```python
from build123d import *

# Parameters (mm, degrees)
SKETCH4_W           = 8
SKETCH4_H           = 5
EXTRUDE1_DEPTH      = 19.1
SKETCH6_W           = 17.706910835
SKETCH6_H           = 1.662230216
CUT_EXTRUDE1_DEPTH  = 18.6
SKETCH7_W           = 17.592020929
SKETCH7_H           = 1.332722913
CUT_EXTRUDE2_DEPTH  = 18.6
SKETCH8_W           = 5.300719424
SKETCH8_H           = 17.765707434
SKETCH8_W_2         = 2.943884892
SKETCH8_H_2         = 17.795443645
CUT_EXTRUDE3_DEPTH  = 18.6
SKETCH10_W          = 3.9
SKETCH10_H          = 17.990453763
CUT_EXTRUDE4_DEPTH  = 2
SKETCH11_R          = 0.25
CUT_EXTRUDE5_DEPTH  = 2
CUT_EXTRUDE6_DEPTH  = 2
SKETCH14_R          = 0.35
CUT_EXTRUDE8_DEPTH  = 2
CUT_EXTRUDE16_DEPTH = 2.6
CUT_EXTRUDE16_DRAFT = 3.5
SKETCH29_W          = 8
SKETCH29_H          = 5
SKETCH29_W_2        = 6
SKETCH29_H_2        = 4.3
CUT_EXTRUDE19_DEPTH = 2.5
CUT_EXTRUDE20_DEPTH = 5.3
CUT_EXTRUDE21_DEPTH = 7
SKETCH19_R          = 1
CUT_EXTRUDE11_DEPTH = 11.25


with BuildPart() as part:
    # Sketch4 → Extrude1 (new body)
    with BuildSketch(Plane.XY):
        with Locations((-4, 2.5)):
            Rectangle(SKETCH4_W, SKETCH4_H)
    extrude(amount=EXTRUDE1_DEPTH)

    # Sketch6 → Cut-Extrude1 (cut)
    with BuildSketch(Plane(origin=(0, 0, 0), x_dir=(0, 0, -1), z_dir=(1, 0, 0))):
        with Locations((-10.453455418, -0.081115108)):
            Rectangle(SKETCH6_W, SKETCH6_H)
    extrude(amount=-CUT_EXTRUDE1_DEPTH, mode=Mode.SUBTRACT)

    # Sketch7 → Cut-Extrude2 (cut)
    with BuildSketch(Plane(origin=(0, 0, 0), x_dir=(0, 0, -1), z_dir=(1, 0, 0))):
        with Locations((-10.396010465, 4.916361457)):
            Rectangle(SKETCH7_W, SKETCH7_H)
    extrude(amount=-CUT_EXTRUDE2_DEPTH, mode=Mode.SUBTRACT)

    # Sketch8 → Cut-Extrude3 (cut)
    with BuildSketch(Plane.XZ.offset(-0.75)):
        with Locations((-9.250359712, 10.482853717)):
            Rectangle(SKETCH8_W, SKETCH8_H)
        with Locations((0.071942446, 10.497721823)):
            Rectangle(SKETCH8_W_2, SKETCH8_H_2)
    extrude(amount=-CUT_EXTRUDE3_DEPTH, mode=Mode.SUBTRACT)

    # Sketch10 → Cut-Extrude4 (cut)
    with BuildSketch(Plane(origin=(0, 4.25, 0), x_dir=(1, 0, 0), z_dir=(0, 1, 0))):
        with Locations((-4, -10.595226882)):
            Rectangle(SKETCH10_W, SKETCH10_H)
    extrude(amount=-CUT_EXTRUDE4_DEPTH, mode=Mode.SUBTRACT)

    # Sketch11 → Cut-Extrude5 (cut)
    with BuildSketch(Plane(origin=(0, 2.25, 0), x_dir=(1, 0, 0), z_dir=(0, 1, 0))):
        with Locations(Location((-3.85, -11.2, 0), (0, 0, 270))):  # turned: the seam where the file's is
            Circle(SKETCH11_R)
    extrude(amount=-CUT_EXTRUDE5_DEPTH, mode=Mode.SUBTRACT)

    # Sketch12 → Cut-Extrude6 (cut)
    with BuildSketch(Plane(origin=(0, 2.25, 0), x_dir=(1, 0, 0), z_dir=(0, 1, 0))):
        with BuildLine():
            Line((-3.2, -19.099584714), (-3.2, -11.099584714))
            ThreePointArc((-3.2, -11.099584714), (-2.95, -10.849584714), (-2.7, -11.099584714))
            Line((-2.7, -11.099584714), (-2.7, -19.099584714))
            ThreePointArc((-2.7, -19.099584714), (-2.95, -19.349584714), (-3.2, -19.099584714))
        make_face()
    extrude(amount=-CUT_EXTRUDE6_DEPTH, mode=Mode.SUBTRACT)

    # Sketch14 → Cut-Extrude8 (cut)
    with BuildSketch(Plane(origin=(0, 2.25, 0), x_dir=(1, 0, 0), z_dir=(0, 1, 0))):
        with Locations(Location((-4.95, -1.975, 0), (0, 0, 270))):  # turned: the seam where the file's is
            Circle(SKETCH14_R)
    extrude(amount=-CUT_EXTRUDE8_DEPTH, mode=Mode.SUBTRACT)


with BuildPart() as cut_extrude16_tool:
    # Sketch28 → Cut-Extrude16 (with draft: the straight prism first)
    with BuildSketch(Plane.XY.offset(1.6)):
        with BuildLine():
            ThreePointArc((-3.25, 3.1), (-3, 2.85), (-2.75, 3.1))
            Line((-2.75, 3.1), (-2.75, 5))
            Line((-2.75, 5), (-3.25, 5))
            Line((-3.25, 5), (-3.25, 3.1))
        make_face()
    extrude(amount=-CUT_EXTRUDE16_DEPTH)
    # Cut-Extrude16: the draft: its side faces are tilted about the plane it starts from
    cut_extrude16_sides = [cut_extrude16_tool.faces().sort_by_distance(p)[0] for p in [
        (-3, 2.85, 0.3),
        (-2.75, 4.05, 0.3),
        (-3, 5, 0.3),
        (-3.25, 4.05, 0.3),
    ]]
    draft(cut_extrude16_sides, Plane.XY.offset(1.6), CUT_EXTRUDE16_DRAFT)


with BuildPart() as part_1:
    add(part.part)

    # Cut-Extrude16: cut by cut_extrude16_tool
    add(cut_extrude16_tool.part, mode=Mode.SUBTRACT)

    # Sketch29 → Cut-Extrude19 (cut)
    with BuildSketch(Plane.XY.offset(1.6)):
        with Locations((-4, 2.5)):
            Rectangle(SKETCH29_W, SKETCH29_H)
        with Locations((-4, 2.5)):
            Rectangle(SKETCH29_W_2, SKETCH29_H_2, mode=Mode.SUBTRACT)
    extrude(amount=-CUT_EXTRUDE19_DEPTH, mode=Mode.SUBTRACT)

    # Sketch18 → Cut-Extrude20 (cut, through all)
    with BuildSketch(Plane(origin=(0, 4.65, 0), x_dir=(1, 0, 0), z_dir=(0, 1, 0))):
        Polygon((-3.8, 0), (-7, -0.85), (-7, 0), align=None)
        Polygon((-2.2, 0), (-1, 0), (-1, -0.85), align=None)
    extrude(amount=-CUT_EXTRUDE20_DEPTH, mode=Mode.SUBTRACT)

    # Sketch30 → Cut-Extrude21 (cut, through all)
    with BuildSketch(Plane.ZY.offset(7)):
        Polygon((0, 3.9), (0.85, 4.65), (0, 4.65), align=None)
        Polygon((0, 2.3), (0.85, 0.35), (0, 0.35), align=None)
    extrude(amount=-CUT_EXTRUDE21_DEPTH, mode=Mode.SUBTRACT)

    # Sketch19 → Cut-Extrude11 (cut)
    with BuildSketch(Plane.XY.offset(1.6)):
        with Locations((-4.85, 3.1)):
            Circle(SKETCH19_R)
    extrude(amount=CUT_EXTRUDE11_DEPTH, mode=Mode.SUBTRACT)


solid = part_1.part
```
The listing builds one solid part. Answer for the finished solid, in the listing's coordinates (mm). A direction names the side the tool comes from. Round coordinates to 2 decimals unless told otherwise and drop trailing zeros. Order: outer loops, then holes, each group sorted by start corner. A loop starts at its lowest first (then second) coordinate and runs counter-clockwise, first axis right, second up. Notation, with made-up numbers: (15.5, 50.5) -> (45.5, 50.5) arc R24 cw to (45.5, 63.5) -> close; hole circle Ø7 at (63.5, -37.5). An arc over 180 degrees is marked (long way). Answer as CSV lines item,"result". Start each with the question number.
(1) Find the intervals of material crossed by probe 1 along X at (y, z) = (4.2, 7.5); probe 2 along X at (y, z) = (1.6, 11.2); probe 3 along X at (y, z) = (1, 17.25), in increasing order. Write a range as from..to.
(2) A tool of negligible diameter and unlimited length cuts with its end or side. For faces 1 (the face through (-6.6, 2, 10)), 2 (the face through (-3.2, 2, 15)), 3 (the face through (-4, 2.25, 10)), from which of +Z, -Z, +X, -X, +Y, -Y can it reach the whole face along a straight path? Write none if from no direction.
(3) Flat-ended cylindrical pins translate along their axes: pin 1 Ø0.8 at (y, z) = (2, 16) entering from -X; pin 2 Ø0.5 at (x, z) = (-1.5, 12.5) entering from +Y; pin 3 Ø0.6 at (y, z) = (3.5, 7) entering from +X. Find the tip coordinate at first contact, or state that the pin passes through.
(4) The part is cut by section D-D (x = -4.95). Determine the outline of the cut face in (y, z) (3 decimals).
(5) For a pull along X with two mould halves and no side action, classify faces 4 (the face through (-2, 2, 19.1)), 5 (the face through (-3.3, 3.9, 0.8)), 6 (the face through (-1.458, 2.53, 0.525)), 7 (the face through (-4.9, 2.1, 7.1)) as +X half, -X half, draft (parallel to the pull), parting line (faces both ways), or undercut.
(6) The part is cut by section C-C (y = 1.05). Count the separate pieces of the cut face and the enclosed holes in it, then the cut area to 3 significant figures.
(7) The part is cut by section A-A (z = 13.75). Determine the outline of the cut face in (x, y), then the cut area to 3 significant figures.
(8) The part is cut by section B-B (y = 3.4). Determine the outline of the cut face in (x, z).
Evaluation:
1,probe 1,"-6.6..-5.95, -2.05..-1.4"
1,probe 2,"-6.6..-4.1, -3.6..-3.2, -2.7..-1.4"
1,probe 3,"-6.6..-3.2, -2.7..-1.4"
2,face 1,"+Z, -X, +Y, -Y"
2,face 2,"+Z, +Y, -Y"
2,face 3,"+Z, +Y"
3,pin 1,"x = -6.6"
3,pin 2,"y = 4.25"
3,pin 3,"x = -1.4"
4,outline,"(0.35, 0.85) -> (1.599, 0.305) -> (4.17, 0.305) -> (4.65, 0.85) -> (4.65, 1.6) -> (2.105, 1.6) -> (2.105, 1.625) -> (0.75, 1.625) -> (0.75, 1.6) -> (0.35, 1.6) -> close; (0.75, 2.325) -> (2.105, 2.325) -> (2.105, 12.85) -> (2.25, 12.85) -> (2.25, 19.1) -> (0.75, 19.1) -> close"
5,face 4,"draft"
5,face 5,"undercut"
5,face 6,"+X half"
5,face 7,"undercut"
6,separate pieces,"1"
6,enclosed holes,"2"
6,area,"92.4 mm²"
7,outline,"(-6.6, 0.75) -> (-3.2, 0.75) -> (-3.2, 2.25) -> (-5.95, 2.25) -> (-5.95, 4.25) -> (-6.6, 4.25) -> close; (-2.7, 0.75) -> (-1.4, 0.75) -> (-1.4, 4.25) -> (-2.05, 4.25) -> (-2.05, 2.25) -> (-2.7, 2.25) -> close"
7,area,"9.65 mm²"
8,outline,"(-7, 0.85) -> (-3.8, 0) -> (-3.35, 0) -> (-3.25, 1.6) -> (-5.95, 1.6) -> (-5.95, 19.1) -> (-6.6, 19.1) -> (-6.6, 1.6) -> (-7, 1.6) -> close; (-2.75, 1.6) -> (-2.65, 0) -> (-2.2, 0) -> (-1, 0.85) -> (-1, 1.6) -> (-1.4, 1.6) -> (-1.4, 19.1) -> (-2.05, 19.1) -> (-2.05, 1.6) -> close"
